Design review of the part built by this model. Coordinates are the model's own, in mm. Coordinates: 2 decimals unless noted, no trailing zeros. Write each loop counter-clockwise with the first axis right and the second up, starting at its lowest first coordinate (ties: lowest second). Pieces come first, ordered by that corner, then holes. Notation, with made-up numbers: (35.5, 11) - (49.5, 11) arc R20 ccw to (49.5, 44) - close; hole circle Ø9 at (63.25, -4). An arc over 180 degrees is marked (long way). Use a Markdown table: item, result.
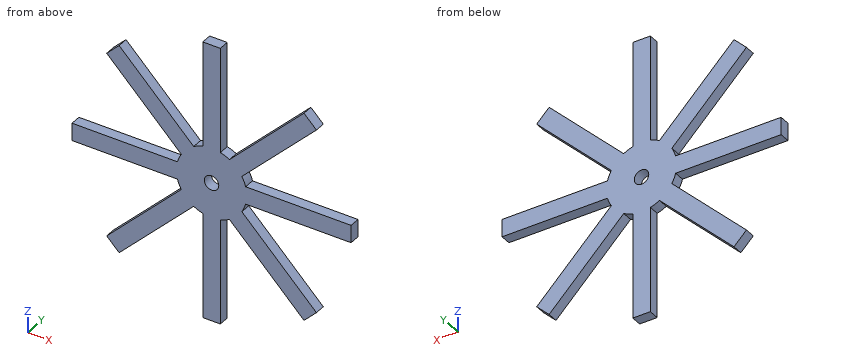
from build123d import *

# Parameters (mm, degrees)
ESBO_O1_R                = 20
ESBO_O1_R_2              = 4.1
RESSALTO_EXTRUS_O1_DEPTH = 6
ESBO_O2_W                = 10
ESBO_O2_H                = 60
ESBO_O2_W_2              = 60
ESBO_O2_H_2              = 10
RESSALTO_EXTRUS_O2_DEPTH = 6


with BuildPart() as part:
    # Esboço1 → Ressalto-extrusão1 (new body)
    with BuildSketch(Plane(origin=(0, 0, 0), x_dir=(1, 0, 0), z_dir=(0, 1, 0))):
        with Locations(Location((0, 0, 0), (0, 0, 270))):
            Circle(ESBO_O1_R)
        with Locations(Location((0, 0, 0), (0, 0, 270))):
            Circle(ESBO_O1_R_2, mode=Mode.SUBTRACT)
    extrude(amount=RESSALTO_EXTRUS_O1_DEPTH)

    # Esboço2 → Ressalto-extrusão2 (add)
    with BuildSketch(Plane(origin=(0, 6, 0), x_dir=(1, 0, 0), z_dir=(0, 1, 0))):
        Polygon((52.583936903, 59.655004715), (59.655004715, 52.583936903), (17.228597844, 10.157530032), (10.157530032, 17.228597844), align=None)
        with Locations((0, 49.364916731)):
            Rectangle(ESBO_O2_W, ESBO_O2_H)
        with Locations((49.364916731, 0)):
            Rectangle(ESBO_O2_W_2, ESBO_O2_H_2)
        Polygon((59.655004715, -52.583936903), (52.583936903, -59.655004715), (10.157530032, -17.228597844), (17.228597844, -10.157530032), align=None)
        with Locations((0, -49.364916731)):
            Rectangle(ESBO_O2_W, ESBO_O2_H)
        Polygon((-52.583936903, -59.655004715), (-59.655004715, -52.583936903), (-17.228597844, -10.157530032), (-10.157530032, -17.228597844), align=None)
        with Locations((-49.364916731, 0)):
            Rectangle(ESBO_O2_W_2, ESBO_O2_H_2)
        Polygon((-59.655004715, 52.583936903), (-52.583936903, 59.655004715), (-10.157530032, 17.228597844), (-17.228597844, 10.157530032), align=None)
    extrude(amount=-RESSALTO_EXTRUS_O2_DEPTH)


solid = part.part
(1) Take a section at A-A on z = 0. Write out the cut boundary in (x, y).
Determined:
| item | result |
|---|---|
| outline | (-79.36, 0) - (-4.1, 0) - (-4.1, 6) - (-79.36, 6) - close; (4.1, 0) - (79.36, 0) - (79.36, 6) - (4.1, 6) - close |
(2) For L1, parallel to Z at x = -39.5, y = 0.45; L2, parallel to X at y = 2.25, z = 0; L3, parallel to Z at x = 22.5, y = 2.35, list the stretches that pass through material, from the lowest coordinate up. Write a range as from..to.
Determined:
| item | result |
|---|---|
| L1 | -46.57..-32.43, -5..5, 32.43..46.57 |
| L2 | -79.36..-4.1, 4.1..79.36 |
| L3 | -29.57..-15.43, -5..5, 15.43..29.57 |
(3) Take a section at D-D on x = -28.5. Write out the cut boundary in (y, z), and give its area (3 significant figures).
Determined:
| item | result |
|---|---|
| outline | (0, -35.57) - (6, -35.57) - (6, -21.43) - (0, -21.43) - close; (0, -5) - (6, -5) - (6, 5) - (0, 5) - close; (0, 21.43) - (6, 21.43) - (6, 35.57) - (0, 35.57) - close |
| area | 230 mm2 |
(4) For pin 1 (5 mm diameter, centred on x = 0, z = 0, fed in from +Y); pin 2 (3 mm diameter, centred on x = -48.5, y = 3.5, fed in from +Z); pin 3 (1.5 mm diameter, centred on y = 2.5, z = 8.5, fed in from -X); pin 4 (1 mm diameter, centred on y = 1, z = 24, fed in from -X), all flat-tipped, find the tip position at first contact; note any pin that passes through.
Determined:
| item | result |
|---|---|
| pin 1 | through |
| pin 2 | z = 57.07 |
| pin 3 | x = -18.44 |
| pin 4 | x = -31.57 |
(5) Take a section at B-B on x = 0. Write out the cut boundary in (y, z).
Determined:
| item | result |
|---|---|
| outline | (0, -79.36) - (6, -79.36) - (6, -4.1) - (0, -4.1) - close; (0, 4.1) - (6, 4.1) - (6, 79.36) - (0, 79.36) - close |
